Geometry: final body of the model. Coordinates: model frame, mm. Coordinates: 2 decimals unless noted, no trailing zeros. Order: outer loops, then holes, each group sorted by start corner. A loop starts at its lowest first (then second) coordinate and runs counter-clockwise, first axis right, second up. Notation, with made-up numbers: M 10.5,51.25 L 69.5,51.25 A17 ccw 69.5,59.25 Z; hole C -17.5,61 d11. An arc over 180 degrees is marked long. Use CSV: the item, a comma, the result in double quotes. Start each with the question number.
Q1. First-contact query: P1, Ø1, axis at y = 1, z = 56.5, coming from the -X side. Flat tip, straight axial feed; report the tip coordinate or a pass-through.
Q2. Section query A-A, the plane y = 0. Output: boundary loops of the cut face in (x, z), and give its area (3 significant figures).
Q3. Section query B-B, the plane x = 0. Output: boundary loops of the cut face in (y, z), and give its area (3 significant figures).
Q4. Ray query, probe 1 along Z at (x, y) = (1.05, 0); probe 2 along X at (y, z) = (0.9, 63.5). Return the intervals inside material, ascending.
Q5. Section query C-C, the plane z = 25.5. Output: boundary loops of the cut face in (x, y), and give its area (3 significant figures).
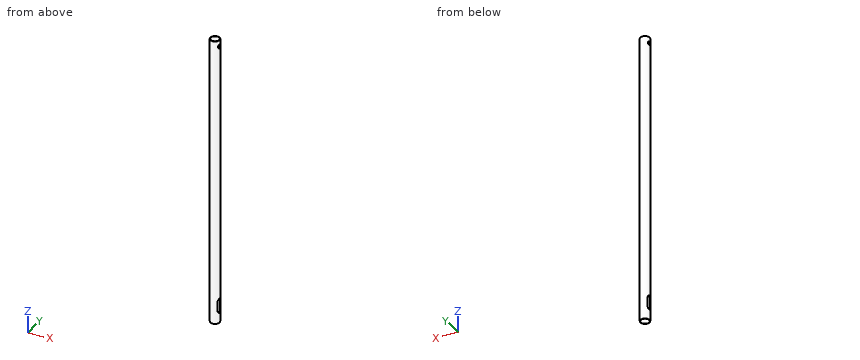
from build123d import *

# Parameters (mm, degrees)
F0_R     = 1.1
F0_R_2   = 1
F1_DEPTH = 69.5
F4_DEPTH = 3.03737
F5_R     = 0.5
F6_DEPTH = 25


with BuildPart() as f1:
    # F0 (on Top) → F1 (new body)
    with BuildSketch(Plane.XY):
        Circle(F0_R)
        Circle(F0_R_2, mode=Mode.SUBTRACT)
    extrude(amount=F1_DEPTH)

    # F3 (on offset) → F4 (cut)
    with BuildSketch(Plane.YZ.offset(-1.1)):
        with BuildLine():
            Line((0.551559, 2.999995), (0.551559, 5.409995))
            ThreePointArc((0.551559, 5.409995), (5e-06, 5.961565), (-0.551559, 5.410005))
            Line((-0.551559, 5.410005), (-0.551559, 3.000005))
            ThreePointArc((-0.551559, 3.000005), (-5e-06, 2.448446), (0.551559, 2.999995))
        make_face()
    extrude(amount=F4_DEPTH, mode=Mode.SUBTRACT)

    # F5 (on offset) → F6 (cut)
    with BuildSketch(Plane.YZ.offset(-1.1)):
        with Locations((0, 68)):
            Circle(F5_R)
    extrude(amount=F6_DEPTH, mode=Mode.SUBTRACT)


solid = f1.part
Responses:
1,P1,"stops at x = -0.98"
2,outline,"M -1.1,0 L -1,0 L -1,2.45 L -1.1,2.45 Z; M -1.1,5.96 L -1,5.96 L -1,67.5 L -1.1,67.5 Z; M -1.1,68.5 L -1,68.5 L -1,69.5 L -1.1,69.5 Z; M 1,0 L 1.1,0 L 1.1,2.45 L 1,2.45 Z; M 1,5.96 L 1.1,5.96 L 1.1,67.5 L 1,67.5 Z; M 1,68.5 L 1.1,68.5 L 1.1,69.5 L 1,69.5 Z"
2,area,"13.0 mm²"
3,outline,"M -1.1,0 L -1,0 L -1,69.5 L -1.1,69.5 Z; M 1,0 L 1.1,0 L 1.1,69.5 L 1,69.5 Z"
3,area,"13.9 mm²"
4,probe 1,"z = 0 to 2.45, 5.96 to 67.5, 68.5 to 69.5"
4,probe 2,"x = -0.63 to -0.44, 0.44 to 0.63"
5,outline,"C 0,0 d2.2; hole C 0,0 d2"
5,area,"0.660 mm²"
